Verification items for the finished model (mm, model axes). Face numbers are marked on the shaded views. Round coordinates to 2 decimals unless told otherwise and drop trailing zeros. Loops run counter-clockwise (first coordinate to the right, second up) from the corner with the lowest first, then second, coordinate; pieces in that order, holes last. Notation, with made-up numbers: (7.25, 57) - (12.25, 57) arc R21 ccw to (12.25, 86) - close; hole circle Ø1 at (77.5, -10). An arc over 180 degrees is marked (long way). Use a Markdown table: item, result. Add a question column.
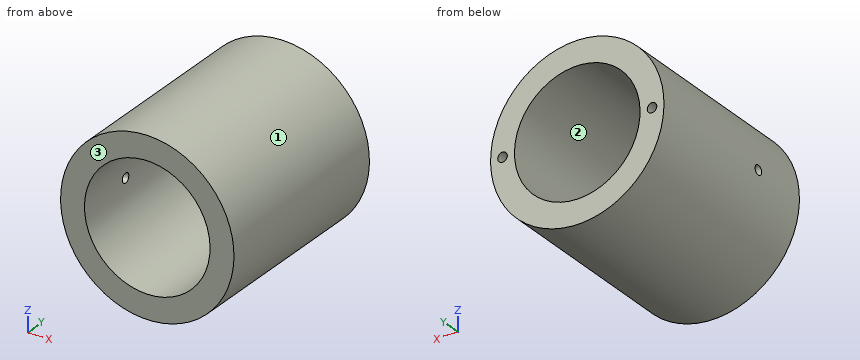
```python
from build123d import *

# Parameters (mm, degrees)
SKETCH_1_R          = 13
SKETCH_1_R_2        = 9.172
EXTRUDE_1_DEPTH     = 25
SKETCH_7_R          = 10.172
CUT_EXTRUDE_2_DEPTH = 50
SKETCH_8_R          = 13
SKETCH_8_R_2        = 10.172
EXTRUDE_2_DEPTH     = 8
SKETCH_11_R         = 10.5
CUT_EXTRUDE_4_DEPTH = 50
EXTRUDE_START       = -33
SKETCH_13_R         = 14.5
SKETCH_13_R_2       = 13
EXTRUDE_3_DEPTH     = 33
SKETCH_4_R          = 0.8
CUT_EXTRUDE_1_DEPTH = 30
SKETCH_10_R         = 0.8
CUT_EXTRUDE_5_DEPTH = 7


with BuildPart() as part:
    # Эскиз1 → Бобышка-Вытянуть1 (new body)
    with BuildSketch(Plane(origin=(0, 0, 0), x_dir=(1, 0, 0), z_dir=(0, 1, 0))):
        with Locations(Location((0, 0, 0), (0, 0, 270))):
            Circle(SKETCH_1_R)
        with Locations(Location((0, 0, 0), (0, 0, 270))):
            Circle(SKETCH_1_R_2, mode=Mode.SUBTRACT)
    extrude(amount=EXTRUDE_1_DEPTH)

    # Эскиз7 → Вырез-Вытянуть2 (cut)
    with BuildSketch(Plane.XZ):
        with Locations(Location((0, 0, 0), (0, 0, 270))):
            Circle(SKETCH_7_R)
    extrude(amount=-CUT_EXTRUDE_2_DEPTH, mode=Mode.SUBTRACT)

    # Эскиз8 → Бобышка-Вытянуть2 (add)
    with BuildSketch(Plane(origin=(0, 25, 0), x_dir=(1, 0, 0), z_dir=(0, 1, 0))):
        with Locations(Location((0, 0, 0), (0, 0, 270))):
            Circle(SKETCH_8_R)
        with Locations(Location((0, 0, 0), (0, 0, 90))):
            Circle(SKETCH_8_R_2, mode=Mode.SUBTRACT)
    extrude(amount=EXTRUDE_2_DEPTH)

    # Эскиз11 → Вырез-Вытянуть4 (cut)
    with BuildSketch(Plane.XZ):
        with Locations(Location((0, 0, 0), (0, 0, 270))):
            Circle(SKETCH_11_R)
    extrude(amount=-CUT_EXTRUDE_4_DEPTH, mode=Mode.SUBTRACT)

    # Эскиз13 → Бобышка-Вытянуть3 (add)
    with BuildSketch(Plane(origin=(0, 33, 0), x_dir=(1, 0, 0), z_dir=(0, 1, 0)).offset(EXTRUDE_START)):
        with Locations(Location((0, 0, 0), (0, 0, 270))):
            Circle(SKETCH_13_R)
        Circle(SKETCH_13_R_2, mode=Mode.SUBTRACT)
    extrude(amount=EXTRUDE_3_DEPTH)

    # Эскиз4 → Вырез-Вытянуть1 (cut)
    with BuildSketch(Plane(origin=(0, 0, 0), x_dir=(0, 0, -1), z_dir=(1, 0, 0))):
        with Locations((0, 10)):
            Circle(SKETCH_4_R)
    extrude(amount=-CUT_EXTRUDE_1_DEPTH, mode=Mode.SUBTRACT)

    # Эскиз10 → Вырез-Вытянуть5 (cut)
    with BuildSketch(Plane(origin=(0, 33, 0), x_dir=(1, 0, 0), z_dir=(0, 1, 0))):
        with Locations(Location((-12.5, 0, 0), (0, 0, 180))):
            Circle(SKETCH_10_R)
        with Locations((12.5, 0)):
            Circle(SKETCH_10_R)
    extrude(amount=-CUT_EXTRUDE_5_DEPTH, mode=Mode.SUBTRACT)


solid = part.part
```
Q1. Section check A-A on z = 0. Record the cut outline in (x, y).
Q2. Release check for a two-part mould opening along Z. For the marked faces 1, 2 and 3 record: +Z half, -Z half, draft (parallel to the pull), parting line (faces both ways), or undercut.
Q3. Go/stop test with flat-tipped pins: pin 1 Ø10 at (x, y) = (-11, 18) entering from +Z; pin 2 Ø5 at (y, z) = (28, -3) entering from -X; pin 3 Ø1.3 at (x, z) = (12.5, 0) entering from +Y. Record where each tip stops, or that it passes through.
Q4. Thickness scan on line 1 along Y through (x, z) = (-12.7, 0); line 2 along X through (y, z) = (9, 0). Record the ranges inside material, lowest first.
Q5. Section check B-B on x = 0. Record the cut outline in (y, z).
Q6. Section check C-C on z = -3.5. Record the cut outline in (x, y).
Q7. Section check D-D on y = 17. Record the cut outline in (x, z), plus the area to 3 significant figures.
Determined:
| question | item | result |
|---|---|---|
| 1 | outline | (-14.5, 0) - (-10.5, 0) - (-10.5, 9.2) - (-14.5, 9.2) - close; (-14.5, 10.8) - (-10.5, 10.8) - (-10.5, 33) - (-11.7, 33) - (-11.7, 26) - (-13.3, 26) - (-13.3, 33) - (-14.5, 33) - close; (10.5, 0) - (14.5, 0) - (14.5, 33) - (13.3, 33) - (13.3, 26) - (11.7, 26) - (11.7, 33) - (10.5, 33) - close |
| 2 | face 1 | parting line |
| 2 | face 2 | undercut |
| 2 | face 3 | draft |
| 3 | pin 1 | stops at z = 13.2 |
| 3 | pin 2 | stops at x = -14.49 |
| 3 | pin 3 | stops at y = 26 |
| 4 | line 1 | y = 0 to 9.2, 10.8 to 26 |
| 4 | line 2 | x = -14.5 to -10.5, 10.5 to 14.5 |
| 5 | outline | (0, -14.5) - (33, -14.5) - (33, -10.5) - (0, -10.5) - close; (0, 10.5) - (33, 10.5) - (33, 14.5) - (0, 14.5) - close |
| 6 | outline | (-14.07, 0) - (-9.9, 0) - (-9.9, 33) - (-14.07, 33) - close; (9.9, 0) - (14.07, 0) - (14.07, 33) - (9.9, 33) - close |
| 7 | outline | circle Ø29 at (0, 0); hole circle Ø21 at (0, 0) |
| 7 | area | 314 mm² |
